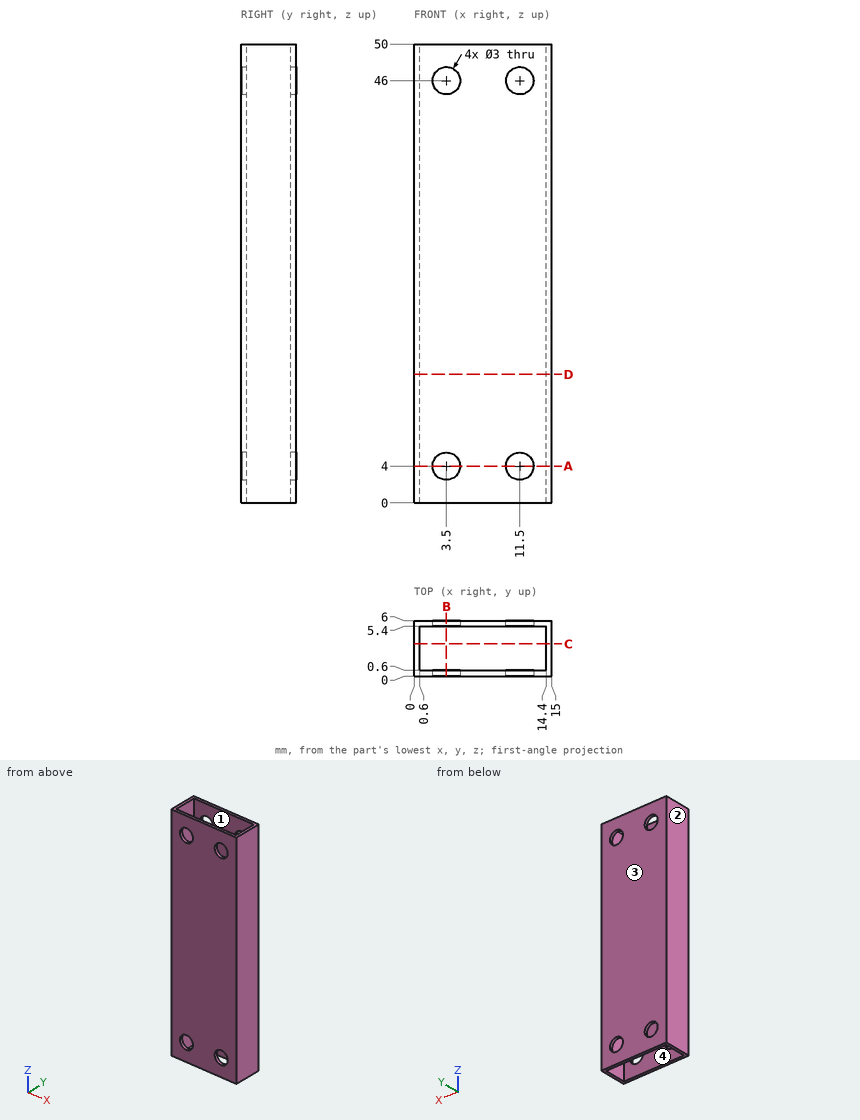
Geometry check sheet. Reference: drawing and pictorial views, mm from the part's lowest x, y, z. Give positions to 0.01 mm unless a question says otherwise; leave off trailing zeros. Order: outer loops, then holes, each group sorted by start corner. A loop starts at its lowest first (then second) coordinate and runs counter-clockwise, first axis right, second up.
1. Section check B-B, the plane x = 3.5. Enter the section's corners in (y, z), and give its area (3 significant figures).
2. Section check A-A, the plane z = 4. Enter the section's corners in (x, y), and give its area (3 significant figures).
3. Gauge pin test, flat end, axial feed: pin 1 Ø2.5 at (x, z) = (3.5, 46) entering from +Y. Record the tip position at first contact, or that the pin passes through.
4. Section check C-C, the plane y = 3.5. Enter the section's corners in (x, z).
5. Thickness scan on L1, parallel to X at y = 0.35, z = 4; L2, parallel to X at y = 1.1, z = 19; L3, parallel to Y at x = 10, z = 35. Record the ranges inside material, lowest first.
6. Release check for a two-part mould opening along X. For the marked faces 1, 2, 3 and 4 record: pulls with the +X half, pulls with the -X half, needs draft (parallel to the pull), parting line crosses it, or undercut.
7. Section check D-D, the plane z = 14. Enter the section's corners in (x, y).
Values follow:
1. outline: (0, 0) - (0.6, 0) - (0.6, 2.5) - (0, 2.5) - close; (0, 5.5) - (0.6, 5.5) - (0.6, 44.5) - (0, 44.5) - close; (0, 47.5) - (0.6, 47.5) - (0.6, 50) - (0, 50) - close; (5.4, 0) - (6, 0) - (6, 2.5) - (5.4, 2.5) - close; (5.4, 5.5) - (6, 5.5) - (6, 44.5) - (5.4, 44.5) - close; (5.4, 47.5) - (6, 47.5) - (6, 50) - (5.4, 50) - close
1. area: 52.8 mm2
2. outline: (0, 0) - (2, 0) - (2, 0.6) - (0.6, 0.6) - (0.6, 5.4) - (2, 5.4) - (2, 6) - (0, 6) - close; (5, 0) - (10, 0) - (10, 0.6) - (5, 0.6) - close; (5, 5.4) - (10, 5.4) - (10, 6) - (5, 6) - close; (13, 0) - (15, 0) - (15, 6) - (13, 6) - (13, 5.4) - (14.4, 5.4) - (14.4, 0.6) - (13, 0.6) - close
2. area: 16.6 mm2
3. pin 1: passes through
4. outline: (0, 0) - (0.6, 0) - (0.6, 50) - (0, 50) - close; (14.4, 0) - (15, 0) - (15, 50) - (14.4, 50) - close
5. L1: x = 0 to 2, 5 to 10, 13 to 15
5. L2: x = 0 to 0.6, 14.4 to 15
5. L3: y = 0 to 0.6, 5.4 to 6
6. face 1: undercut
6. face 2: pulls with the -X half
6. face 3: needs draft
6. face 4: undercut
7. outline: (0, 0) - (15, 0) - (15, 6) - (0, 6) - close; hole (0.6, 0.6) - (14.4, 0.6) - (14.4, 5.4) - (0.6, 5.4) - close
